The listing builds one solid part. Answer for the finished solid, in the listing's coordinates (mm). A direction names the side the tool comes from. Round coordinates to 2 decimals unless told otherwise and drop trailing zeros. Write each loop counter-clockwise with the first axis right and the second up, starting at its lowest first coordinate (ties: lowest second). Pieces come first, ordered by that corner, then holes. Notation, with made-up numbers: (-1.75, 64.25) - (55.25, 64.25) arc R28 cw to (55.25, 97.25) - close; hole circle Ø2 at (10, 31.25). An arc over 180 degrees is marked (long way). Return JSON: item names as keys, results as strings. Group by question number.
(1) Each of these flat-tipped pins is pushed along its axis until it touches: pin 1 (2 mm diameter, centred on x = 100.5, z = -25.5, fed in from +Y); pin 2 (6 mm diameter, centred on y = 246.5, z = -12.5, fed in from +X). Where does it stop, or does it pass through?
(2) Section C-C, the plane x = -16 is taken. Write down the section's boundary in (y, z), then the cut area to 3 significant figures.
(3) Section B-B, the plane z = 0 is taken. Write down the section's boundary in (x, y), then the cut area to 3 significant figures.
(4) Which of the six approach directions +Z, -Z, +X, -X, +Y, -Y give full straight-line access (tool end or side, diameter ignored) to faces 1 (the flat face through (-195, 193, 2)), 2 (the flat face through (-3, 182, 195))?
(5) Determine the mould class of faces 3 (the cylindrical face through (205.14, 281.728, 4.166)), 4 (the flat face through (-3, 0, -3)), 5 (the flat face through (-3, 20, -2)), 6 (the flat face through (-3, 182, -195)) for opening direction Y: +Y half, -Y half, draft (parallel to the pull), parting line (faces both ways), or undercut.
(6) Section A-A, the plane y = 34 is taken. Write down the section's boundary in (x, z).
(7) Section D-D, the plane y = 250 is taken. Write down the section's boundary in (x, z), then the cut area to 3 significant figures.
(8) Find the intervals of material crossed by line 1 along Y through (x, z) = (209, 0); line 2 along Z through (x, y) = (40.5, 347.5); line 3 along X through (y, z) = (109.5, -72.5), in increasing order. Write a range as [from, to].
```python
from build123d import *

# Parameters (mm, degrees)
SKETCH1_W           = 430
SKETCH1_H           = 390
BOSS_EXTRUDE1_DEPTH = 370
SHELL1_T            = -20
CUT_EXTRUDE2_REACH  = 601.854
SKETCH2_R           = 32


with BuildPart() as part:
    # Sketch1 → Boss-Extrude1 (new body)
    with BuildSketch(Plane(origin=(0, 0, 0), x_dir=(1, 0, 0), z_dir=(0, 1, 0))):
        Rectangle(SKETCH1_W, SKETCH1_H)
    extrude(amount=BOSS_EXTRUDE1_DEPTH)

    # Shell1
    shell1_openings = [part.faces().sort_by_distance(p)[0] for p in [
        (0, 370, 0),
    ]]
    offset(amount=SHELL1_T, openings=shell1_openings, kind=Kind.INTERSECTION)

    # Sketch2 → Cut-Extrude2 (cut, up to next)
    with BuildSketch(Plane(origin=(215, 0, 0), x_dir=(0, 0, -1), z_dir=(1, 0, 0)), mode=Mode.PRIVATE) as cut_extrude2_sk1:
        with Locations((0, 250)):
            Circle(SKETCH2_R)
    cut_extrude2_tool1 = extrude(cut_extrude2_sk1.sketch, amount=-CUT_EXTRUDE2_REACH, mode=Mode.PRIVATE) & part.part
    add(cut_extrude2_tool1.solids().sort_by_distance((215, 250, 0))[0], mode=Mode.SUBTRACT)


solid = part.part
```
Working result:
{
 "1": {"pin 1": "stops at y = 20", "pin 2": "stops at x = -195"},
 "2": {"outline": "(0, -195) - (370, -195) - (370, -175) - (20, -175) - (20, 175) - (370, 175) - (370, 195) - (0, 195) - close", "area": "21,800 mm^2"},
 "3": {"outline": "(-215, 0) - (215, 0) - (215, 218) - (195, 218) - (195, 20) - (-195, 20) - (-195, 370) - (-215, 370) - close; (195, 282) - (215, 282) - (215, 370) - (195, 370) - close", "area": "21,300 mm^2"},
 "4": {"face 1": "+Y", "face 2": "+Z, +X, -X, +Y, -Y"},
 "5": {"face 3": "undercut", "face 4": "-Y half", "face 5": "+Y half", "face 6": "draft"},
 "6": {"outline": "(-215, -195) - (215, -195) - (215, 195) - (-215, 195) - close; hole (-195, -175) - (195, -175) - (195, 175) - (-195, 175) - close"},
 "7": {"outline": "(-215, -195) - (215, -195) - (215, -32) - (195, -32) - (195, -175) - (-195, -175) - (-195, 175) - (195, 175) - (195, 32) - (215, 32) - (215, 195) - (-215, 195) - close", "area": "29,900 mm^2"},
 "8": {"line 1": "y = [0, 218], [282, 370]", "line 2": "z = [-195, -175], [175, 195]", "line 3": "x = [-215, -195], [195, 215]"}
}
